Drawing for the job (mm, zero at the part's lowest x, y, z). Give positions to 0.01 mm unless a question says otherwise; leave off trailing zeros. Write each loop counter-clockwise with the first axis right and the second up, starting at its lowest first coordinate (ties: lowest second). Pieces come first, ordered by that corner, then holes. Notation, with made-up numbers: M 2,80 L 29,80 A13 cw 29,103 Z; hole C 0,34 d3. An arc over 180 degrees is marked long. Write item = value, one per line. Start each with the question number.
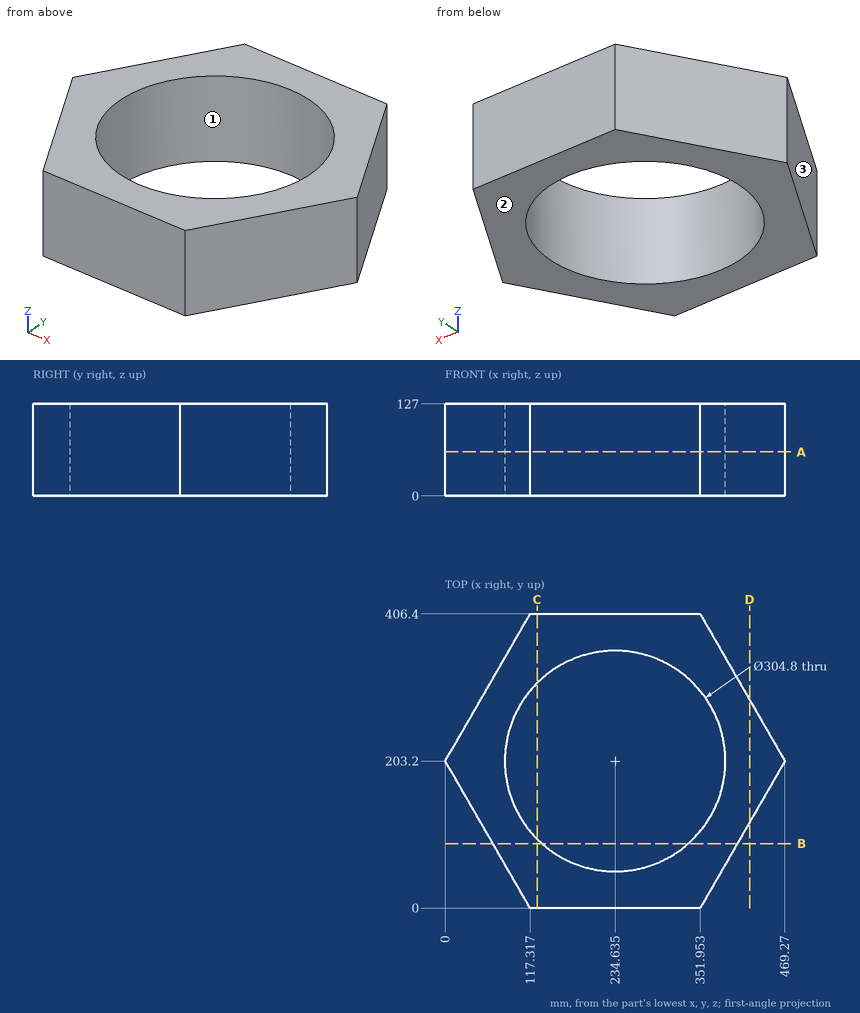
Q1. Two-plate mould, pull along X, no slides. Class the marked faces 1, 2 and 3: +X half, -X half, draft (parallel to the pull), parting line (faces both ways), or undercut.
Q2. Probe line 1 along Y through (x, z) = (210, 5) (1 decimal); line 2 along Y through (x, z) = (229.5, 118.5); line 3 along X through (y, z) = (109.5, 75.5) (1 decimal). List the from-to ranges inside material, lowest first.
Q3. Slice it at A-A (z = 61). Give the cut face in (x, y) (1 decimal).
Q4. Drop flat-ended pins along their axis: P1, Ø6, axis at y = 298.5, z = 62.5, coming from the +X side; P2, Ø8, axis at y = 177, z = 18.5, coming from the -X side. Give the stop position or say it passes through.
Q5. Slice it at B-B (y = 89). Give the cut face in (x, z), and give its area (3 significant figures).
Q6. Slice it at C-C (x = 127). Give the cut face in (y, z), and give its area (3 significant figures).
Q7. Slice it at D-D (x = 420.5). Give the cut face in (y, z), and give its area (3 significant figures).
Working result:
q1.face_1 = undercut
q1.face_2 = draft
q1.face_3 = -X half
q2.line_1 = 0 to 52.8, 353.6 to 406.4
q2.line_2 = 0 to 50.89, 355.51 to 406.4
q2.line_3 = 54.1 to 114.4, 354.8 to 415.2
q3.outline = M 0,203.2 L 117.3,0 L 352,0 L 469.3,203.2 L 352,406.4 L 117.3,406.4 Z; hole C 234.6,203.2 d304.8
q4.P1 = 415.98
q4.P2 = 12.82
q5.outline = M 65.93,0 L 133.72,0 L 133.72,127 L 65.93,127 Z; M 335.55,0 L 403.34,0 L 403.34,127 L 335.55,127 Z
q5.area = 17,200 mm2
q6.outline = M 0,0 L 95.31,0 L 95.31,127 L 0,127 Z; M 311.09,0 L 406.4,0 L 406.4,127 L 311.09,127 Z
q6.area = 24,200 mm2
q7.outline = M 118.73,0 L 287.67,0 L 287.67,127 L 118.73,127 Z
q7.area = 21,500 mm2
